Geometry check sheet. Reference: the model listing, model coordinates, mm. Face numbers are marked on the shaded views. A direction names the side the tool comes from. Give positions to 0.01 mm unless a question says otherwise; leave off trailing zeros. Write each loop counter-clockwise with the first axis right and the second up, starting at its lowest first coordinate (ties: lowest second). Pieces come first, ordered by that corner, then holes. Notation, with made-up numbers: M 18.5,-34.5 L 62.5,-34.5 A24 cw 62.5,-7.5 Z; hole C -19.5,54 d4. An arc over 180 degrees is marked long. Use one line per item in the form item = value. Start each with the question number.
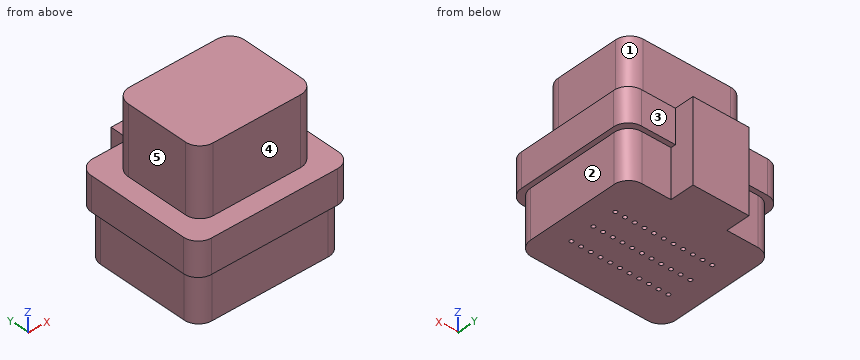
```python
from build123d import *

# Parameters (mm, degrees)
SKETCH_1_W          = 32
SKETCH_1_H          = 27
EXTRUDE_1_DEPTH     = 7
SKETCH_2_W          = 24
SKETCH_2_H          = 19
EXTRUDE_2_DEPTH     = 14
SKETCH_3_W          = 30
SKETCH_3_H          = 25
EXTRUDE_3_DEPTH     = 10
FILLET_1_R          = 3
SKETCH_4_W          = 11.544617985
SKETCH_4_H          = 17
EXTRUDE_4_DEPTH     = 5
SKETCH_5_R          = 0.4
CUT_EXTRUDE_1_DEPTH = 1


with BuildPart() as part:
    # ｽｹｯﾁ1 → ﾎﾞｽ - 押し出し1 (new body)
    with BuildSketch(Plane.XY):
        with Locations((16, 13.5)):
            Rectangle(SKETCH_1_W, SKETCH_1_H)
    extrude(amount=EXTRUDE_1_DEPTH)

    # ｽｹｯﾁ2 → ﾎﾞｽ - 押し出し2 (add)
    with BuildSketch(Plane.XY.offset(7)):
        with Locations((16, 13.5)):
            Rectangle(SKETCH_2_W, SKETCH_2_H)
    extrude(amount=EXTRUDE_2_DEPTH)

    # ｽｹｯﾁ3 → ﾎﾞｽ - 押し出し3 (add)
    with BuildSketch(Plane(origin=(0, 0, 0), x_dir=(-1, 0, 0), z_dir=(0, 0, -1))):
        with Locations((-16, 13.5)):
            Rectangle(SKETCH_3_W, SKETCH_3_H)
    extrude(amount=EXTRUDE_3_DEPTH)

    # ﾌｨﾚｯﾄ1
    fillet_1_edges = [part.edges().sort_by_distance(p)[0] for p in [
        (28, 23, 14),
        (4, 23, 14),
        (4, 4, 14),
        (28, 4, 14),
        (31, 1, -5),
        (1, 1, -5),
        (1, 26, -5),
        (31, 26, -5),
        (0, 27, 3.5),
        (32, 27, 3.5),
        (32, 0, 3.5),
        (0, 0, 3.5),
    ]]
    fillet(fillet_1_edges, radius=FILLET_1_R)

    # ｽｹｯﾁ4 → ﾎﾞｽ - 押し出し4 (add)
    with BuildSketch(Plane(origin=(0, 26, 0), x_dir=(1, 0, 0), z_dir=(0, 1, 0))):
        with Locations((16.191136059, 1.5)):
            Rectangle(SKETCH_4_W, SKETCH_4_H)
    extrude(amount=EXTRUDE_4_DEPTH)

    # ｽｹｯﾁ5 → ｶｯﾄ - 押し出し1 (cut)
    with BuildSketch(Plane(origin=(0, 0, -10), x_dir=(-1, 0, 0), z_dir=(0, 0, -1))):
        with Locations((-16.191136059, 13)):
            Circle(SKETCH_5_R)
        with Locations((-14.191136059, 13)):
            Circle(SKETCH_5_R)
        with Locations((-12.191136059, 13)):
            Circle(SKETCH_5_R)
        with Locations((-10.191136059, 13)):
            Circle(SKETCH_5_R)
        with Locations((-8.191136059, 13)):
            Circle(SKETCH_5_R)
        with Locations((-6.191136059, 13)):
            Circle(SKETCH_5_R)
        with Locations((-16.191136059, 18)):
            Circle(SKETCH_5_R)
        with Locations((-14.191136059, 18)):
            Circle(SKETCH_5_R)
        with Locations((-12.191136059, 18)):
            Circle(SKETCH_5_R)
        with Locations((-10.191136059, 18)):
            Circle(SKETCH_5_R)
        with Locations((-8.191136059, 18)):
            Circle(SKETCH_5_R)
        with Locations((-6.191136059, 18)):
            Circle(SKETCH_5_R)
        with Locations((-16.191136059, 8)):
            Circle(SKETCH_5_R)
        with Locations((-14.191136059, 8)):
            Circle(SKETCH_5_R)
        with Locations((-12.191136059, 8)):
            Circle(SKETCH_5_R)
        with Locations((-10.191136059, 8)):
            Circle(SKETCH_5_R)
        with Locations((-8.191136059, 8)):
            Circle(SKETCH_5_R)
        with Locations((-6.191136059, 8)):
            Circle(SKETCH_5_R)
        with Locations((-26.191136059, 18)):
            Circle(SKETCH_5_R)
        with Locations((-24.191136059, 18)):
            Circle(SKETCH_5_R)
        with Locations((-22.191136059, 18)):
            Circle(SKETCH_5_R)
        with Locations((-20.191136059, 18)):
            Circle(SKETCH_5_R)
        with Locations((-18.191136059, 13)):
            Circle(SKETCH_5_R)
        with Locations((-20.191136059, 13)):
            Circle(SKETCH_5_R)
        with Locations((-22.191136059, 13)):
            Circle(SKETCH_5_R)
        with Locations((-24.191136059, 13)):
            Circle(SKETCH_5_R)
        with Locations((-26.191136059, 13)):
            Circle(SKETCH_5_R)
        with Locations((-26.191136059, 8)):
            Circle(SKETCH_5_R)
        with Locations((-24.191136059, 8)):
            Circle(SKETCH_5_R)
        with Locations((-22.191136059, 8)):
            Circle(SKETCH_5_R)
        with Locations((-20.191136059, 8)):
            Circle(SKETCH_5_R)
        with Locations((-18.191136059, 8)):
            Circle(SKETCH_5_R)
        with Locations((-18.191136059, 18)):
            Circle(SKETCH_5_R)
    extrude(amount=-CUT_EXTRUDE_1_DEPTH, mode=Mode.SUBTRACT)


solid = part.part
```
(1) Sectioned sample at D-D, the plane y = 25. Record the boundary of the cut face in (x, z).
(2) Depth check by flat-ended pin: pin 1 (0.6 mm diameter, centred on x = 10, y = 18, fed in from -Z); pin 2 (15.5 mm diameter, centred on x = 15.5, z = 16, fed in from +Y); pin 3 (1.5 mm diameter, centred on x = 19, z = 11, fed in from -Y); pin 4 (2.5 mm diameter, centred on y = 29, z = 1, fed in from +X). Enter the tip coordinate at first touch or a pass-through.
(3) Tool access check on the marked faces 1, 2, 3, 4 and 5. Record the directions out of +Z, -Z, +X, -X, +Y, -Y that give a thin tool (end or side, any length) a straight path to the whole face; none if there is none.
(4) Thickness scan on probe 1 along Y at (x, z) = (16.5, 19); probe 2 along Z at (x, y) = (18, 27.5); probe 3 along Z at (x, y) = (6, 8). Record the ranges inside material, lowest first. Write a range as [from, to].
(5) Sectioned sample at A-A, the plane z = 10.5. Record the boundary of the cut face in (x, y), plus the area to 3 significant figures.
(6) Sectioned sample at C-C, the plane z = 4. Record the boundary of the cut face in (x, y), plus the area to 3 significant figures.
(7) Sectioned sample at B-B, the plane y = 17. Record the boundary of the cut face in (x, z), plus the area to 3 significant figures.
Numbers:
q1.outline = M 0.17,0 L 1.76,0 L 1.76,-10 L 30.24,-10 L 30.24,0 L 31.83,0 L 31.83,7 L 0.17,7 Z
q2.pin_1 = -10
q2.pin_2 = 23
q2.pin_3 = 4
q2.pin_4 = 21.96
q3.face_1 = +Z, +X, +Y
q3.face_2 = -Z, +X, +Y, -Y
q3.face_3 = +Z, -Z, +X, +Y
q3.face_4 = +Z, +X, -X, -Y
q3.face_5 = +Z, -X, +Y, -Y
q4.probe_1 = [4, 23]
q4.probe_2 = [-10, 7]
q4.probe_3 = [-9, 21]
q5.outline = M 4,7 A3 ccw 7,4 L 25,4 A3 ccw 28,7 L 28,20 A3 ccw 25,23 L 7,23 A3 ccw 4,20 Z
q5.area = 448 mm2
q6.outline = M 0,3 A3 ccw 3,0 L 29,0 A3 ccw 32,3 L 32,24 A3 ccw 29,27 L 21.96,27 L 21.96,31 L 10.42,31 L 10.42,27 L 3,27 A3 ccw 0,24 Z
q6.area = 902 mm2
q7.outline = M 0,0 L 1,0 L 1,-10 L 31,-10 L 31,0 L 32,0 L 32,7 L 28,7 L 28,21 L 4,21 L 4,7 L 0,7 Z
q7.area = 860 mm2
